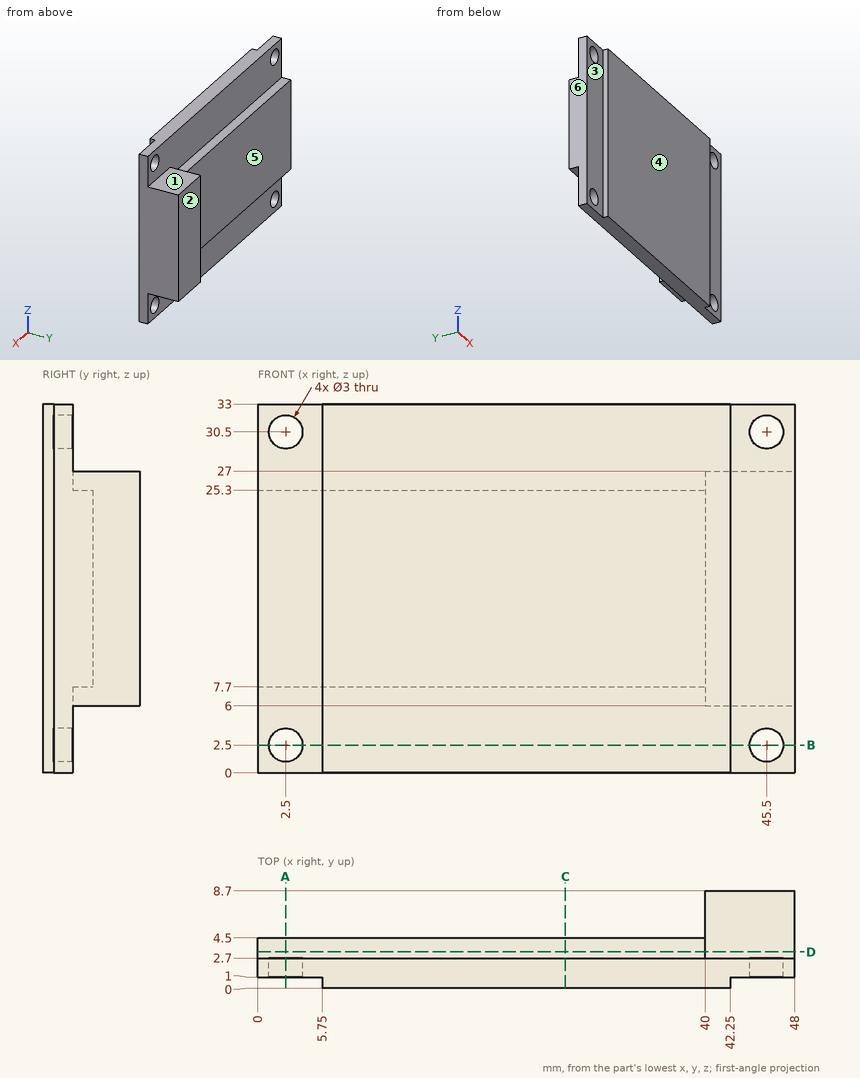
Drawing for the job (mm, zero at the part's lowest x, y, z). A direction names the side the tool comes from. Give positions to 0.01 mm unless a question says otherwise; leave off trailing zeros. Write each loop counter-clockwise with the first axis right and the second up, starting at its lowest first coordinate (ties: lowest second). Pieces come first, ordered by that corner, then holes. Notation, with made-up numbers: M 61.25,-23 L 96.25,-23 A34 ccw 96.25,8 Z; hole C 19.5,-6.5 d10. An arc over 180 degrees is marked long. Use CSV: the item, a comma, the result in double quotes.
Item 1: Drill centre lines: probe 1 along Y at (x, z) = (6, 7); probe 2 along X at (y, z) = (7.5, 17); probe 3 along Z at (x, y) = (3.5, 3.25). Where is each one in solid material? Low to high.
Taken from the geometry:
probe 1,"y = 0 to 2.7"
probe 2,"x = 40 to 48"
probe 3,"z = 7.7 to 25.3"
Item 2: Slice it at B-B on z = 2.5. Write the cut outline in (x, y), plus the area to 3 significant figures.
Taken from the geometry:
outline,"M 0,1 L 1,1 L 1,2.7 L 0,2.7 Z; M 4,1 L 5.75,1 L 5.75,0 L 42.25,0 L 42.25,1 L 44,1 L 44,2.7 L 4,2.7 Z; M 47,1 L 48,1 L 48,2.7 L 47,2.7 Z"
area,"108 mm²"
Item 3: Slice it at D-D on y = 3.25. Write the cut outline in (x, z), plus the area to 3 significant figures.
Taken from the geometry:
outline,"M 0,7.7 L 40,7.7 L 40,6 L 48,6 L 48,27 L 40,27 L 40,25.3 L 0,25.3 Z"
area,"872 mm²"
Item 4: Pin check, flat tips, straight feed: P1, Ø1.1, axis at y = 0.5, z = 22.5, coming from the +X side; P2, Ø4, axis at x = 33, z = 30, coming from the +Y side; P3, Ø1.4, axis at x = 29.5, y = 3.5, coming from the -Z side; P4, Ø2, axis at y = 6.5, z = 7, coming from the -X side. Stop position of each tip, or through.
Taken from the geometry:
P1,"stops at x = 48"
P2,"stops at y = 2.7"
P3,"stops at z = 7.7"
P4,"stops at x = 40"
Item 5: Slice it at A-A on x = 2.5. Write the cut outline in (y, z), plus the area to 3 significant figures.
Taken from the geometry:
outline,"M 1,0 L 2.7,0 L 2.7,1 L 1,1 Z; M 1,4 L 2.7,4 L 2.7,7.7 L 4.5,7.7 L 4.5,25.3 L 2.7,25.3 L 2.7,29 L 1,29 Z; M 1,32 L 2.7,32 L 2.7,33 L 1,33 Z"
area,"77.6 mm²"
Item 6: Pull direction Y, two halves, no side cores. Call the marked faces 4, 5 and 6: +Y half, -Y half, draft (parallel to the pull), parting line (faces both ways), or undercut.
Taken from the geometry:
face 4,"-Y half"
face 5,"+Y half"
face 6,"draft"
Item 7: Slice it at C-C on x = 27.5. Write the cut outline in (y, z).
Taken from the geometry:
outline,"M 0,0 L 2.7,0 L 2.7,7.7 L 4.5,7.7 L 4.5,25.3 L 2.7,25.3 L 2.7,33 L 0,33 Z"
Item 8: Which spindle directions (+Z, -Z, +X, -X, +Y, -Y) get a long thin tool onto all of the face, cutting with end or side? Do the marked faces 1, 2 and 3. Say none if no direction does.
Taken from the geometry:
face 1,"+Z, +X, -X, +Y"
face 2,"+Z, -Z, +X, -X, +Y"
face 3,"+Z, -Z, -X, -Y"
